Build history of the part. All positions in model axes, mm. A direction names the side the tool comes from. Round coordinates to 2 decimals unless told otherwise and drop trailing zeros. Loops run counter-clockwise (first coordinate to the right, second up) from the corner with the lowest first, then second, coordinate; pieces in that order, holes last. Notation, with made-up numbers: M 7,36 L 41,36 A21 cw 41,69 Z; hole C 3,20.5 d4. An arc over 180 degrees is marked long. One line per item, written item: value.
```python
from build123d import *

# Parameters (mm, degrees)
SKETCH_2_R      = 5.25
EXTRUDE_1_DEPTH = 0.8
EXTRUDE_2_DEPTH = 3.5
SKETCH_4_R      = 2.5
EXTRUDE_3_DEPTH = 16
FILLET_1_R      = 1
CHAMFER_1_SIZE  = 0.5


with BuildPart() as part:
    # Эскиз2 → Бобышка-Вытянуть1 (new body)
    with BuildSketch(Plane.XY):
        Circle(SKETCH_2_R)
    extrude(amount=EXTRUDE_1_DEPTH)

    # Эскиз3 → Бобышка-Вытянуть2 (add)
    with BuildSketch(Plane.XY.offset(0.8)):
        Polygon((-2.309401077, 4), (-4.618802154, 0), (-2.309401077, -4), (2.309401077, -4), (4.618802154, 0), (2.309401077, 4), align=None)
    extrude(amount=EXTRUDE_2_DEPTH)

    # Эскиз4 → Бобышка-Вытянуть3 (add)
    with BuildSketch(Plane(origin=(0, 0, 0), x_dir=(-1, 0, 0), z_dir=(0, 0, -1))):
        Circle(SKETCH_4_R)
    extrude(amount=EXTRUDE_3_DEPTH)

    # Скругление1
    fillet_1_edges = [part.edges().sort_by_distance(p)[0] for p in [
        (0, 4, 4.3),
        (-3.464101615, 2, 4.3),
        (-3.464101615, -2, 4.3),
        (0, -4, 4.3),
        (3.464101615, -2, 4.3),
        (3.464101615, 2, 4.3),
    ]]
    fillet(fillet_1_edges, radius=FILLET_1_R)

    # Фаска1
    chamfer_1_edges = [part.edges().sort_by_distance(p)[0] for p in [
        (2.5, 0, -16),
    ]]
    chamfer(chamfer_1_edges, length=CHAMFER_1_SIZE)


solid = part.part
```
Item 1: Drop flat-ended pins along their axis: P1, Ø1, axis at x = -1, z = 0, coming from the -Y side; P2, Ø6, axis at x = -2.5, z = -1, coming from the +Y side; P3, Ø0.8, axis at x = 0.5, z = 1.5, coming from the +Y side; P4, Ø1.3, axis at x = 0.5, z = 2.5, coming from the -Y side. Give the stop position or say it passes through.
Check values:
P1: stops at y = -5.23
P2: stops at y = 5.25
P3: stops at y = 4
P4: stops at y = -4
Item 2: Which spindle directions (+Z, -Z, +X, -X, +Y, -Y) get a long thin tool onto all of the face, cutting with end or side? Do faces 1 (the face through (-3.48, -1.97, 2.03)), 2 (the face through (0.54, -2.44, -7.64)), 3 (the face through (0, 4, 2)), 4 (the face through (3.448, -2.028, 2.033)), 5 (the face through (3.48, 1.97, 2.03)). Say none if no direction does.
Check values:
face 1: +Z, -X, -Y
face 2: -Z
face 3: +Z, +X, -X, +Y
face 4: +Z, +X, -Y
face 5: +Z, +X, +Y
Item 3: Slice it at C-C, the plane z = 2.75. Give the cut face in (x, y), and give its area (3 significant figures).
Check values:
outline: M -4.62,0 L -2.31,-4 L 2.31,-4 L 4.62,0 L 2.31,4 L -2.31,4 Z
area: 55.4 mm2
Item 4: Wall check: line 1 along Z through (x, y) = (-3.5, 2.5); line 2 along Y through (x, z) = (0.5, 1.5); line 3 along Y through (x, z) = (-1.5, -1.25). Give the ranges that are in metal, low to high.
Check values:
line 1: z = 0 to 0.8
line 2: y = -4 to 4
line 3: y = -2 to 2
Item 5: Slice it at B-B, the plane z = -2.75. Give the cut face in (x, y).
Check values:
outline: C 0,0 d5
Item 6: Slice it at A-A, the plane x = 0. Give the cut face in (y, z).
Check values:
outline: M -5.25,0 L -2.5,0 L -2.5,-15.5 L -2,-16 L 2,-16 L 2.5,-15.5 L 2.5,0 L 5.25,0 L 5.25,0.8 L 4,0.8 L 4,3.3 A1 ccw 3,4.3 L -3,4.3 A1 ccw -4,3.3 L -4,0.8 L -5.25,0.8 Z
